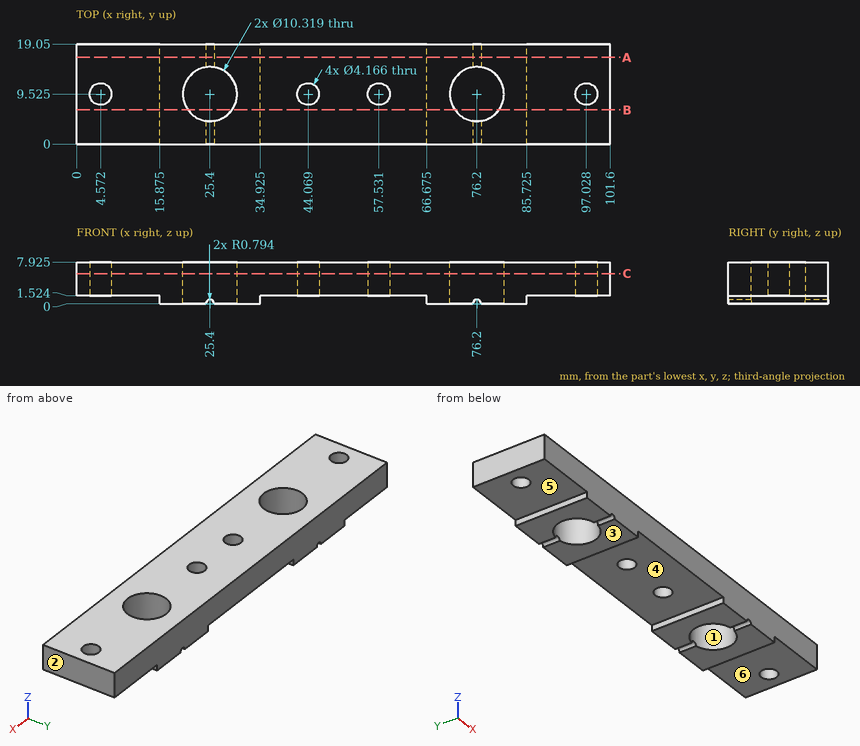
Part print with two shaded views. Sizes in mm from the minimum x, y, z corner. A direction names the side the tool comes from. Coordinates: 2 decimals unless noted, no trailing zeros. Loops run counter-clockwise (first coordinate to the right, second up) from the corner with the lowest first, then second, coordinate; pieces in that order, holes last. Notation, with made-up numbers: M 55.5,9.25 L 92.5,9.25 A37 ccw 92.5,48.25 Z; hole C 19.25,86.5 d6. An arc over 180 degrees is marked long. Use CSV: the item, a comma, the result in double quotes. Start each with the question number.
1. Probe probe 1 along X at (y, z) = (12, 7.25); probe 2 along X at (y, z) = (6.75, 5); probe 3 along Z at (x, y) = (36, 4) (1 decimal). List the from-to ranges inside material, lowest first. Write a range as [from, to].
2. Flat gauge pins, fed straight in: pin 1 (0.5 mm diameter, centred on y = 12.5, z = 0.5, fed in from -X) (3 decimals); pin 2 (9.5 mm diameter, centred on x = 44, y = 14, fed in from -Z); pin 3 (0.8 mm diameter, centred on y = 10, z = 1, fed in from +X) (3 decimals). Where does each tip first touch, or does it go through?
3. Tool access for the marked faces 4, 5 and 6: list every direction of +Z, -Z, +X, -X, +Y, -Y with a clear straight run to the whole face (end or side of a thin tool).
4. Band-saw the part on C-C, the plane z = 5.75. Give the number of separate pieces and of enclosed holes in the cut face, then the cut area to 3 significant figures.
5. Two-plate mould, pull along X, no slides. Class the marked faces 1, 2 and 3: pulls with the +X half, pulls with the -X half, needs draft (parallel to the pull), parting line crosses it, or undercut.
6. Band-saw the part on A-A, the plane y = 16.5. List the corners of the cut face in (x, z) (1 decimal).
7. Band-saw the part on B-B, the plane y = 6.5. List the corners of the cut face in (x, z) (1 decimal), then the cut area to 3 significant figures.
Entries:
1,probe 1,"x = [0, 20.87], [29.93, 71.67], [80.73, 101.6]"
1,probe 2,"x = [0, 21.05], [29.75, 71.85], [80.55, 101.6]"
1,probe 3,"z = [1.5, 7.9]"
2,pin 1,"stops at x = 15.875"
2,pin 2,"stops at z = 1.52"
2,pin 3,"stops at x = 85.725"
3,face 4,"-Z, +Y, -Y"
3,face 5,"-Z, -X, +Y, -Y"
3,face 6,"-Z, +X, +Y, -Y"
4,separate pieces,"1"
4,enclosed holes,"6"
4,area,"1,710 mm2"
5,face 1,"undercut"
5,face 2,"pulls with the +X half"
5,face 3,"needs draft"
6,outline,"M 0,1.5 L 15.9,1.5 L 15.9,0 L 24.6,0 A0.8 cw 26.2,0 L 34.9,0 L 34.9,1.5 L 66.7,1.5 L 66.7,0 L 75.4,0 A0.8 cw 77,0 L 85.7,0 L 85.7,1.5 L 101.6,1.5 L 101.6,7.9 L 0,7.9 Z"
7,outline,"M 0,1.5 L 15.9,1.5 L 15.9,0 L 21.2,0 L 21.2,7.9 L 0,7.9 Z; M 29.6,0 L 34.9,0 L 34.9,1.5 L 66.7,1.5 L 66.7,0 L 72,0 L 72,7.9 L 29.6,7.9 Z; M 80.4,0 L 85.7,0 L 85.7,1.5 L 101.6,1.5 L 101.6,7.9 L 80.4,7.9 Z"
7,area,"576 mm2"
